Check sheet for the modelled part. Datum: model origin and axes. Units: mm. A direction names the side the tool comes from. Give positions to 0.01 mm unless a question says otherwise; leave off trailing zeros. Write each loop counter-clockwise with the first axis right and the second up, starting at its lowest first coordinate (ties: lowest second). Pieces come first, ordered by that corner, then holes. Notation, with made-up numbers: M -25.5,-5 L -18.5,-5 A25 ccw -18.5,34 Z; hole C 37.25,64.25 d4. An arc over 180 degrees is marked long. Write item = value, one per line. Start each with the question number.
1) Cross-section at B-B, the plane y = 66.5. Record the cut outline in (x, z), plus the area to 3 significant figures.
2) Cross-section at D-D, the plane x = 58. Record the cut outline in (y, z), plus the area to 3 significant figures.
3) Go/stop test with flat-tipped pins: pin 1 (7.5 mm diameter, centred on x = 30.5, y = 69, fed in from +Z); pin 2 (1 mm diameter, centred on x = 25, z = 37, fed in from -Y); pin 3 (12 mm diameter, centred on x = 19, y = 72, fed in from -Z); pin 4 (11.5 mm diameter, centred on x = 48.56, z = 15, fed in from -Y). Record where each tip stops, or that it passes through.
4) Scan lines: line 1 along X through (y, z) = (16, 15); line 2 along X through (y, z) = (75.5, 44); line 3 along Z through (x, y) = (29, 75). Record each from-to range of solid material in increasing order. Write a range as [from, to].
5) Cross-section at C-C, the plane z = 15. Record the cut outline in (x, y), plus the area to 3 significant figures.
6) Mould release check, pull along Z, two halves, no side actions. Record for faces 1 (the cylindrical face through (10.411, 72.363, 18.381)), 2 (the flat face through (24, 72, 27)), 3 (the flat face through (24, 67, 10)): released by +Z, released by -Z, zero draft, split by the parting line, or undercut.
7) Access from +Z, -Z, +X, -X, +Y, -Y to the whole of each face (thin tool, end or side, straight path). Record for faces 4 (the flat face through (45, 19.581, 10)), 5 (the flat face through (24, 72, 33)), 6 (the flat face through (33.565, 17, 30)), 7 (the flat face through (23, 67, 50)).
8) Cross-section at A-A, the plane z = 35. Record the cut outline in (x, y), plus the area to 3 significant figures.
```python
from build123d import *

# Parameters (mm, degrees)
SKETCH1_W                  = 30
SKETCH1_H                  = 5
BOSS_EXTRUDE1_DEPTH        = 60
FILLET1_R                  = 10
F_10_0_10_DIAMETER_HOLE1_D = 10
SKETCH4_W                  = 50
SKETCH4_H                  = 6
BOSS_EXTRUDE4_DEPTH        = 40
CUT_EXTRUDE3_DEPTH         = 40
BOSS_EXTRUDE5_DEPTH        = 20
BOSS_EXTRUDE5_DEPTH_BACK   = 5
F_5_0_5_DIAMETER_HOLE1_D   = 5
CUT_EXTRUDE4_DEPTH         = 108.392141664
FILLET2_R                  = 5
FILLET3_R                  = 5


with BuildPart() as part:
    # Sketch1 → Boss-Extrude1 (new body)
    with BuildSketch(Plane.XY):
        with Locations((48.564868256, 17.080601224)):
            Rectangle(SKETCH1_W, SKETCH1_H)
    extrude(amount=BOSS_EXTRUDE1_DEPTH)

    # Fillet1
    fillet1_edges = [part.edges().sort_by_distance(p)[0] for p in [
        (63.564868256, 17.080601224, 60),
        (63.564868256, 17.080601224, 0),
    ]]
    fillet(fillet1_edges, radius=FILLET1_R)

    # Ø10.0 (10) Diameter Hole1 (through all)
    with Locations(Plane(origin=(48.564868256, 19.580601224, 15), x_dir=(0, 0, 1), z_dir=(0, 1, 0))):
        with Locations((0, 0), (30, 0)):
            Hole(F_10_0_10_DIAMETER_HOLE1_D / 2)

    # Sketch4 → Boss-Extrude4 (add)
    with BuildSketch(Plane(origin=(0, 19.580601224, 0), x_dir=(1, 0, 0), z_dir=(0, 1, 0))):
        with Locations((38.564868256, -30)):
            Rectangle(SKETCH4_W, SKETCH4_H)
    extrude(amount=BOSS_EXTRUDE4_DEPTH)

    # Sketch10 → Cut-Extrude3 (cut)
    with BuildSketch(Plane.XY.offset(33)):
        Polygon((33.564868256, 19.580601224), (13.564868256, 59.580601224), (13.564868256, 19.580601224), align=None)
        Polygon((63.564868256, 59.580601224), (43.564868256, 59.580601224), (63.564868256, 19.580601224), align=None)
    extrude(amount=-CUT_EXTRUDE3_DEPTH, mode=Mode.SUBTRACT)

    # Sketch11 → Boss-Extrude5 (add, two sides: drawn at the far end of the back side and taken through both)
    with BuildSketch(Plane(origin=(0, 59.580601224, 0), x_dir=(1, 0, 0), z_dir=(0, 1, 0)).offset(-BOSS_EXTRUDE5_DEPTH_BACK)):
        Polygon((43.564868256, -30), (43.564868256, -10), (3.564868256, -10), (3.564868256, -50), (43.564868256, -50), align=None)
    extrude(amount=BOSS_EXTRUDE5_DEPTH + BOSS_EXTRUDE5_DEPTH_BACK)

    # Ø5.0 (5) Diameter Hole1 (through all)
    with Locations(Plane(origin=(36.564868256, 74.580601224, 50), x_dir=(1, 0, 0), z_dir=(0, 0, 1))):
        with Locations((0, 0), (-25, 0)):
            Hole(F_5_0_5_DIAMETER_HOLE1_D / 2)

    # Sketch15 → Cut-Extrude4 (cut, through all)
    with BuildSketch(Plane(origin=(43.564868256, 0, 0), x_dir=(0, 0, -1), z_dir=(1, 0, 0))):
        Polygon((-30, 64.580601224), (-27, 64.580601224), (-27, 79.580601224), (-33, 79.580601224), (-33, 64.580601224), align=None)
    extrude(amount=-CUT_EXTRUDE4_DEPTH, mode=Mode.SUBTRACT)

    # Fillet2
    fillet2_edges = [part.edges().sort_by_distance(p)[0] for p in [
        (43.564868256, 79.580601224, 41.5),
    ]]
    fillet(fillet2_edges, radius=FILLET2_R)

    # Fillet3
    fillet3_edges = [part.edges().sort_by_distance(p)[0] for p in [
        (43.564868256, 79.580601224, 18.5),
    ]]
    fillet(fillet3_edges, radius=FILLET3_R)


solid = part.part
```
Reply:
q1.outline = M 3.56,10 L 43.56,10 L 43.56,27 L 3.56,27 Z; M 3.56,33 L 43.56,33 L 43.56,50 L 3.56,50 Z
q1.area = 1,360 mm2
q2.outline = M 14.58,1.04 L 19.58,1.04 L 19.58,27 L 30.71,27 L 30.71,33 L 19.58,33 L 19.58,58.96 L 14.58,58.96 Z
q2.area = 356 mm2
q3.pin_1 = 50
q3.pin_2 = 54.58
q3.pin_3 = 10
q3.pin_4 = 14.58
q4.line_1 = [33.56, 43.56], [53.56, 63.56]
q4.line_2 = [3.56, 9.24], [13.89, 34.24], [38.89, 43.48]
q4.line_3 = [10, 27], [33, 50]
q5.outline = M 3.56,54.58 L 43.56,54.58 L 43.56,74.58 A5 ccw 38.56,79.58 L 3.56,79.58 Z; M 33.56,14.58 L 43.56,14.58 L 43.56,19.58 L 33.56,19.58 Z; M 53.56,14.58 L 63.56,14.58 L 63.56,19.58 L 53.56,19.58 Z; hole C 11.56,74.58 d5; hole C 36.56,74.58 d5
q5.area = 1,060 mm2
q6.face_1 = zero draft
q6.face_2 = undercut
q6.face_3 = released by -Z
q7.face_4 = -Z, +X, -X
q7.face_5 = +X, -X, +Y
q7.face_6 = +Z, -Z, -X, -Y
q7.face_7 = +Z, +X, -X, +Y
q8.outline = M 3.56,54.58 L 43.56,54.58 L 43.56,74.58 A5 ccw 38.56,79.58 L 3.56,79.58 Z; M 33.56,14.58 L 63.56,14.58 L 63.56,19.58 L 33.56,19.58 Z; hole C 11.56,74.58 d5; hole C 36.56,74.58 d5
q8.area = 1,110 mm2
